Drawing for the job (mm, zero at the part's lowest x, y, z). A direction names the side the tool comes from. Give positions to 0.01 mm unless a question says otherwise; leave off trailing zeros. Order: outer loops, then holes, each group sorted by start corner. A loop starts at its lowest first (then second) coordinate and runs counter-clockwise, first axis right, second up. Notation, with made-up numbers: (-5, 84.5) - (7, 84.5) arc R33 ccw to (7, 121.5) - close; hole circle Ø1 at (3, 39). An arc over 180 degrees is marked (long way). One line per item, written item: value.
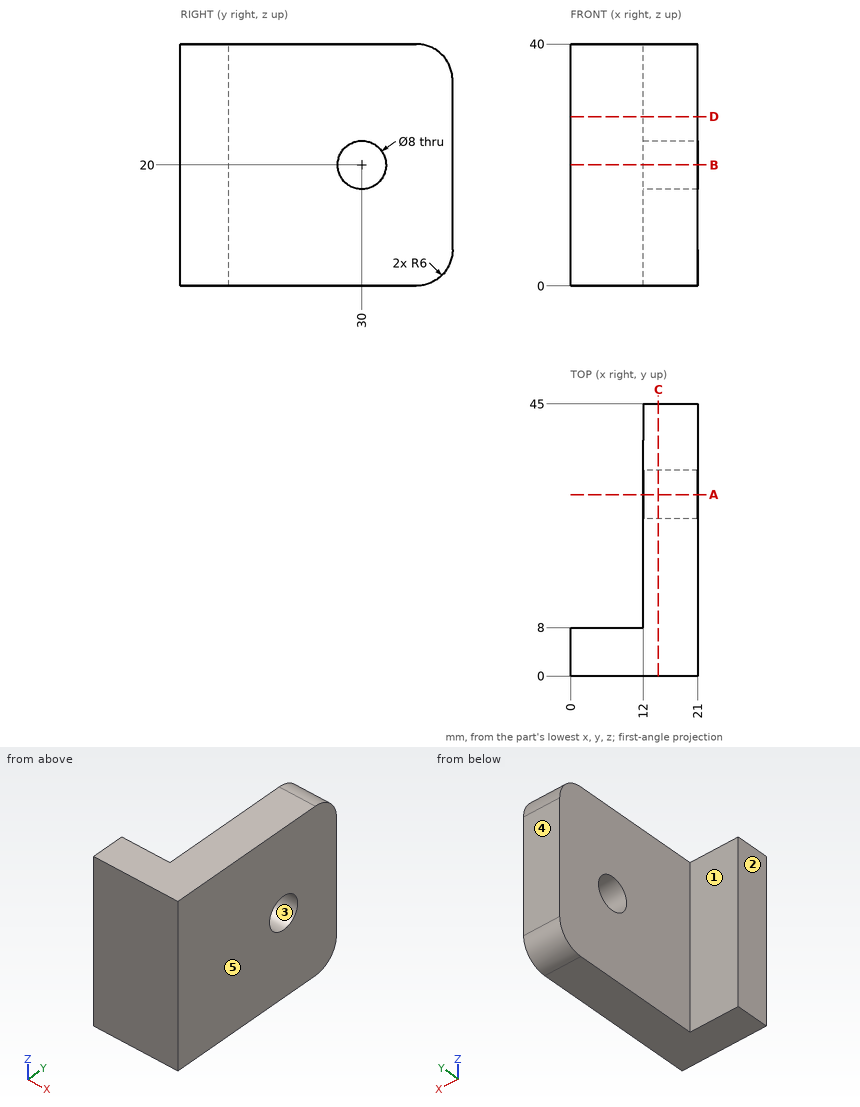
1) Cut at D-D, the plane z = 28. Give the cut face in (x, y), then the cut area to 3 significant figures.
Outcome:
outline: (0, 0) - (21, 0) - (21, 45) - (12, 45) - (12, 8) - (0, 8) - close
area: 501 mm^2
2) Cut at C-C, the plane x = 14.5. Give the cut face in (y, z), then the cut area to 3 significant figures.
Outcome:
outline: (0, 0) - (39, 0) arc R6 ccw to (45, 6) - (45, 34) arc R6 ccw to (39, 40) - (0, 40) - close; hole circle Ø8 at (30, 20)
area: 1,730 mm^2
3) Mould opens along Y. For the marked faces 3, 4 and 5 say: released by +Y, released by -Y, zero draft, split by the parting line, or undercut.
Outcome:
face 3: undercut
face 4: released by +Y
face 5: zero draft
4) Cut at B-B, the plane z = 20. Give the cut face in (x, y), then the cut area to 3 significant figures.
Outcome:
outline: (0, 0) - (21, 0) - (21, 26) - (12, 26) - (12, 8) - (0, 8) - close; (12, 34) - (21, 34) - (21, 45) - (12, 45) - close
area: 429 mm^2
5) Cut at A-A, the plane y = 30. Give the cut face in (x, z).
Outcome:
outline: (12, 0) - (21, 0) - (21, 16) - (12, 16) - close; (12, 24) - (21, 24) - (21, 40) - (12, 40) - close
6) Pin check, flat tips, straight feed: pin 1 (9.5 mm diameter, centred on x = 4.5, z = 20, fed in from +Y); pin 2 (4 mm diameter, centred on y = 21.5, z = 5, fed in from -X). Stop position of each tip, or through.
Outcome:
pin 1: stops at y = 8
pin 2: stops at x = 12
7) Which spindle directions (+Z, -Z, +X, -X, +Y, -Y) get a long thin tool onto all of the face, cutting with end or side? Do the marked faces 1 and 2. Say none if no direction does.
Outcome:
face 1: +Z, -Z, -X, +Y
face 2: +Z, -Z, -X, +Y, -Y
8) Drill centre lines: line 1 along Y through (x, z) = (14.5, 20); line 2 along X through (y, z) = (9, 8.5); line 3 along Y through (x, z) = (2.25, 36.5). Where is each one in solid material? Low to high. Write a range as from..to.
Outcome:
line 1: y = 0..26, 34..45
line 2: x = 12..21
line 3: y = 0..8
